Could you check a few things on this model? Use its own coordinates, in mm. A direction names the side the tool comes from. Coordinates: 2 decimals unless noted, no trailing zeros. Order: outer loops, then holes, each group sorted by start corner. A loop starts at its lowest first (then second) coordinate and runs counter-clockwise, first axis right, second up. Notation, with made-up numbers: (9.25, 65.25) - (27.25, 65.25) arc R33 cw to (27.25, 98.25) - close; hole circle Ø7 at (-14.5, 74). An arc over 180 degrees is marked (long way). Answer as a JSON object with one key per item and string values. Group by question number.
(1) Will these pins go through, and if not, where does the flat tip stop? P1, Ø2, axis at x = -14.5, y = 11.5, coming from the +Z side; P2, Ø5, axis at x = 33.5, z = 35.5, coming from the +Y side; P3, Ø7, axis at x = -33.5, z = -33.5, coming from the -Y side.
(2) We'd pull the mould along X, two halves only. Please class faces 4 (the flat face through (-1, 4, 42.5)), 5 (the flat face through (-42.5, 4, 1)), 6 (the flat face through (36.1, 4.166, -34.3)): pulls with the +X half, pulls with the -X half, needs draft (parallel to the pull), parting line crosses it, or undercut.
(3) Imagine slicing it at B-B, the plane x = -33.5. Write out the boundary of the cut face in (y, z), and give its area (3 significant figures).
(4) Please list where these lines run through material, in increasing order: probe 1 along Z at (x, y) = (33.5, 7); probe 2 along Z at (x, y) = (33.5, 8.25).
(5) Imagine slicing it at A-A, the plane z = 33.5. Write out the boundary of the cut face in (x, y), and give its area (3 significant figures).
(6) Which directions (+Z, -Z, +X, -X, +Y, -Y) give clear straight access to the entire face, cutting with the end or side of a thin tool? Please do faces 1 (the flat face through (-14.5, 4, -40)), 2 (the flat face through (-32.7, 4.166, 30.9)), 3 (the flat face through (0, 10, -15)).
from build123d import *

# Parameters (mm, degrees)
SKETCH1_W           = 85
SKETCH1_H           = 85
SKETCH1_R           = 2.4575
BOSS_EXTRUDE1_DEPTH = 8
SKETCH2_R           = 3.969
CUT_EXTRUDE1_DEPTH  = 4.166
SKETCH3_R           = 5
SKETCH3_R_2         = 2.4575
BOSS_EXTRUDE2_DEPTH = 3.5
BOSS_EXTRUDE3_DEPTH = 5
SKETCH5_W           = 29
SKETCH5_H           = 8
CUT_EXTRUDE2_DEPTH  = 10
FILLET1_R           = 2.5
CUT_EXTRUDE3_REACH  = 59.5


with BuildPart() as part:
    # Sketch1 → Boss-Extrude1 (new body)
    with BuildSketch(Plane(origin=(0, 0, 0), x_dir=(1, 0, 0), z_dir=(0, 1, 0))):
        Rectangle(SKETCH1_W, SKETCH1_H)
        with Locations((-33.5, 33.5)):
            Circle(SKETCH1_R, mode=Mode.SUBTRACT)
        with Locations((-33.5, -33.5)):
            Circle(SKETCH1_R, mode=Mode.SUBTRACT)
        with Locations((33.5, -33.5)):
            Circle(SKETCH1_R, mode=Mode.SUBTRACT)
        with Locations((33.5, 33.5)):
            Circle(SKETCH1_R, mode=Mode.SUBTRACT)
    extrude(amount=BOSS_EXTRUDE1_DEPTH)

    # Sketch2 → Cut-Extrude1 (cut)
    with BuildSketch(Plane.XZ):
        with Locations((-33.5, 33.5)):
            Circle(SKETCH2_R)
        with Locations((33.5, 33.5)):
            Circle(SKETCH2_R)
        with Locations((33.5, -33.5)):
            Circle(SKETCH2_R)
        with Locations((-33.5, -33.5)):
            Circle(SKETCH2_R)
    extrude(amount=-CUT_EXTRUDE1_DEPTH, mode=Mode.SUBTRACT)

    # Sketch3 → Boss-Extrude2 (add)
    with BuildSketch(Plane(origin=(0, 8, 0), x_dir=(1, 0, 0), z_dir=(0, 1, 0))):
        with Locations((33.5, -33.5)):
            Circle(SKETCH3_R)
        with Locations((33.5, -33.5)):
            Circle(SKETCH3_R_2, mode=Mode.SUBTRACT)
        with Locations((-33.5, -33.5)):
            Circle(SKETCH3_R)
        with Locations((-33.5, -33.5)):
            Circle(SKETCH3_R_2, mode=Mode.SUBTRACT)
        with Locations((-33.5, 33.5)):
            Circle(SKETCH3_R)
        with Locations((-33.5, 33.5)):
            Circle(SKETCH3_R_2, mode=Mode.SUBTRACT)
        with Locations((33.5, 33.5)):
            Circle(SKETCH3_R)
        with Locations((33.5, 33.5)):
            Circle(SKETCH3_R_2, mode=Mode.SUBTRACT)
    extrude(amount=BOSS_EXTRUDE2_DEPTH)

    # Sketch4 → Boss-Extrude3 (add)
    with BuildSketch(Plane(origin=(0, 8, 0), x_dir=(1, 0, 0), z_dir=(0, 1, 0))):
        with BuildLine():
            Line((2.2929, -14.5), (2.2929, -13.7071))
            ThreePointArc((2.2929, -13.7071), (2.000006781, -12.999993219), (1.2929, -12.7071))
            Line((1.2929, -12.7071), (-1.2929, -12.7071))
            ThreePointArc((-1.2929, -12.7071), (-2.000006781, -12.999993219), (-2.2929, -13.7071))
            Line((-2.2929, -13.7071), (-2.2929, -14.5))
            ThreePointArc((-2.2929, -14.5), (-2.439346609, -14.853553391), (-2.7929, -15))
            Line((-2.7929, -15), (-14.5, -15))
            ThreePointArc((-14.5, -15), (-14.853553391, -14.853553391), (-15, -14.5))
            Line((-15, -14.5), (-15, 14.5))
            ThreePointArc((-15, 14.5), (-14.853553391, 14.853553391), (-14.5, 15))
            Line((-14.5, 15), (14.5, 15))
            ThreePointArc((14.5, 15), (14.853553391, 14.853553391), (15, 14.5))
            Line((15, 14.5), (15, -14.5))
            ThreePointArc((15, -14.5), (14.853553391, -14.853553391), (14.5, -15))
            Line((14.5, -15), (2.7929, -15))
            ThreePointArc((2.7929, -15), (2.439346609, -14.853553391), (2.2929, -14.5))
        make_face()
    extrude(amount=BOSS_EXTRUDE3_DEPTH)

    # Sketch5 → Cut-Extrude2 (cut)
    with BuildSketch(Plane(origin=(0, 8, 0), x_dir=(1, 0, 0), z_dir=(0, 1, 0))):
        with Locations((0, 38.5)):
            Rectangle(SKETCH5_W, SKETCH5_H)
    extrude(amount=-CUT_EXTRUDE2_DEPTH, mode=Mode.SUBTRACT)

    # Fillet1
    fillet1_edges = [part.edges().sort_by_distance(p)[0] for p in [
        (14.5, 4, -34.5),
        (-14.5, 4, -34.5),
    ]]
    fillet(fillet1_edges, radius=FILLET1_R)

    # Sketch7 → Cut-Extrude3 (cut, up to next)
    with BuildSketch(Plane(origin=(0, 0, -15), x_dir=(-1, 0, 0), z_dir=(0, 0, -1)), mode=Mode.PRIVATE) as cut_extrude3_sk1:
        Polygon((-14.5, 13), (-14.125, 12.38), (-13.75, 13), align=None)
    cut_extrude3_tool1 = extrude(cut_extrude3_sk1.sketch, amount=-CUT_EXTRUDE3_REACH, mode=Mode.PRIVATE) & part.part
    add(cut_extrude3_tool1.solids().sort_by_distance((14.125, 12.793333, -15))[0], mode=Mode.SUBTRACT)
    # Sketch7 → Cut-Extrude3 (cut, up to next)
    with BuildSketch(Plane(origin=(0, 0, -15), x_dir=(-1, 0, 0), z_dir=(0, 0, -1)), mode=Mode.PRIVATE) as cut_extrude3_sk2:
        Polygon((-12.5, 13), (-12.125, 12.38), (-11.75, 13), align=None)
    cut_extrude3_tool2 = extrude(cut_extrude3_sk2.sketch, amount=-CUT_EXTRUDE3_REACH, mode=Mode.PRIVATE) & part.part
    add(cut_extrude3_tool2.solids().sort_by_distance((12.125, 12.793333, -15))[0], mode=Mode.SUBTRACT)
    # Sketch7 → Cut-Extrude3 (cut, up to next)
    with BuildSketch(Plane(origin=(0, 0, -15), x_dir=(-1, 0, 0), z_dir=(0, 0, -1)), mode=Mode.PRIVATE) as cut_extrude3_sk3:
        Polygon((-10.5, 13), (-10.125, 12.38), (-9.75, 13), align=None)
    cut_extrude3_tool3 = extrude(cut_extrude3_sk3.sketch, amount=-CUT_EXTRUDE3_REACH, mode=Mode.PRIVATE) & part.part
    add(cut_extrude3_tool3.solids().sort_by_distance((10.125, 12.793333, -15))[0], mode=Mode.SUBTRACT)
    # Sketch7 → Cut-Extrude3 (cut, up to next)
    with BuildSketch(Plane(origin=(0, 0, -15), x_dir=(-1, 0, 0), z_dir=(0, 0, -1)), mode=Mode.PRIVATE) as cut_extrude3_sk4:
        Polygon((-8.5, 13), (-8.125, 12.38), (-7.75, 13), align=None)
    cut_extrude3_tool4 = extrude(cut_extrude3_sk4.sketch, amount=-CUT_EXTRUDE3_REACH, mode=Mode.PRIVATE) & part.part
    add(cut_extrude3_tool4.solids().sort_by_distance((8.125, 12.793333, -15))[0], mode=Mode.SUBTRACT)
    # Sketch7 → Cut-Extrude3 (cut, up to next)
    with BuildSketch(Plane(origin=(0, 0, -15), x_dir=(-1, 0, 0), z_dir=(0, 0, -1)), mode=Mode.PRIVATE) as cut_extrude3_sk5:
        Polygon((-6.5, 13), (-6.125, 12.38), (-5.75, 13), align=None)
    cut_extrude3_tool5 = extrude(cut_extrude3_sk5.sketch, amount=-CUT_EXTRUDE3_REACH, mode=Mode.PRIVATE) & part.part
    add(cut_extrude3_tool5.solids().sort_by_distance((6.125, 12.793333, -15))[0], mode=Mode.SUBTRACT)
    # Sketch7 → Cut-Extrude3 (cut, up to next)
    with BuildSketch(Plane(origin=(0, 0, -15), x_dir=(-1, 0, 0), z_dir=(0, 0, -1)), mode=Mode.PRIVATE) as cut_extrude3_sk6:
        Polygon((-4.5, 13), (-4.125, 12.38), (-3.75, 13), align=None)
    cut_extrude3_tool6 = extrude(cut_extrude3_sk6.sketch, amount=-CUT_EXTRUDE3_REACH, mode=Mode.PRIVATE) & part.part
    add(cut_extrude3_tool6.solids().sort_by_distance((4.125, 12.793333, -15))[0], mode=Mode.SUBTRACT)
    # Sketch7 → Cut-Extrude3 (cut, up to next)
    with BuildSketch(Plane(origin=(0, 0, -15), x_dir=(-1, 0, 0), z_dir=(0, 0, -1)), mode=Mode.PRIVATE) as cut_extrude3_sk7:
        Polygon((-2.5, 13), (-2.125, 12.38), (-1.75, 13), align=None)
    cut_extrude3_tool7 = extrude(cut_extrude3_sk7.sketch, amount=-CUT_EXTRUDE3_REACH, mode=Mode.PRIVATE) & part.part
    add(cut_extrude3_tool7.solids().sort_by_distance((2.125, 12.793333, -15))[0], mode=Mode.SUBTRACT)
    # Sketch7 → Cut-Extrude3 (cut, up to next)
    with BuildSketch(Plane(origin=(0, 0, -15), x_dir=(-1, 0, 0), z_dir=(0, 0, -1)), mode=Mode.PRIVATE) as cut_extrude3_sk8:
        Polygon((-0.5, 13), (-0.125, 12.38), (0.25, 13), align=None)
    cut_extrude3_tool8 = extrude(cut_extrude3_sk8.sketch, amount=-CUT_EXTRUDE3_REACH, mode=Mode.PRIVATE) & part.part
    add(cut_extrude3_tool8.solids().sort_by_distance((0.125, 12.793333, -15))[0], mode=Mode.SUBTRACT)
    # Sketch7 → Cut-Extrude3 (cut, up to next)
    with BuildSketch(Plane(origin=(0, 0, -15), x_dir=(-1, 0, 0), z_dir=(0, 0, -1)), mode=Mode.PRIVATE) as cut_extrude3_sk9:
        Polygon((1.5, 13), (1.875, 12.38), (2.25, 13), align=None)
    cut_extrude3_tool9 = extrude(cut_extrude3_sk9.sketch, amount=-CUT_EXTRUDE3_REACH, mode=Mode.PRIVATE) & part.part
    add(cut_extrude3_tool9.solids().sort_by_distance((-1.875, 12.793333, -15))[0], mode=Mode.SUBTRACT)
    # Sketch7 → Cut-Extrude3 (cut, up to next)
    with BuildSketch(Plane(origin=(0, 0, -15), x_dir=(-1, 0, 0), z_dir=(0, 0, -1)), mode=Mode.PRIVATE) as cut_extrude3_sk10:
        Polygon((3.5, 13), (3.875, 12.38), (4.25, 13), align=None)
    cut_extrude3_tool10 = extrude(cut_extrude3_sk10.sketch, amount=-CUT_EXTRUDE3_REACH, mode=Mode.PRIVATE) & part.part
    add(cut_extrude3_tool10.solids().sort_by_distance((-3.875, 12.793333, -15))[0], mode=Mode.SUBTRACT)
    # Sketch7 → Cut-Extrude3 (cut, up to next)
    with BuildSketch(Plane(origin=(0, 0, -15), x_dir=(-1, 0, 0), z_dir=(0, 0, -1)), mode=Mode.PRIVATE) as cut_extrude3_sk11:
        Polygon((5.5, 13), (5.875, 12.38), (6.25, 13), align=None)
    cut_extrude3_tool11 = extrude(cut_extrude3_sk11.sketch, amount=-CUT_EXTRUDE3_REACH, mode=Mode.PRIVATE) & part.part
    add(cut_extrude3_tool11.solids().sort_by_distance((-5.875, 12.793333, -15))[0], mode=Mode.SUBTRACT)
    # Sketch7 → Cut-Extrude3 (cut, up to next)
    with BuildSketch(Plane(origin=(0, 0, -15), x_dir=(-1, 0, 0), z_dir=(0, 0, -1)), mode=Mode.PRIVATE) as cut_extrude3_sk12:
        Polygon((7.5, 13), (7.875, 12.38), (8.25, 13), align=None)
    cut_extrude3_tool12 = extrude(cut_extrude3_sk12.sketch, amount=-CUT_EXTRUDE3_REACH, mode=Mode.PRIVATE) & part.part
    add(cut_extrude3_tool12.solids().sort_by_distance((-7.875, 12.793333, -15))[0], mode=Mode.SUBTRACT)
    # Sketch7 → Cut-Extrude3 (cut, up to next)
    with BuildSketch(Plane(origin=(0, 0, -15), x_dir=(-1, 0, 0), z_dir=(0, 0, -1)), mode=Mode.PRIVATE) as cut_extrude3_sk13:
        Polygon((9.5, 13), (9.875, 12.38), (10.25, 13), align=None)
    cut_extrude3_tool13 = extrude(cut_extrude3_sk13.sketch, amount=-CUT_EXTRUDE3_REACH, mode=Mode.PRIVATE) & part.part
    add(cut_extrude3_tool13.solids().sort_by_distance((-9.875, 12.793333, -15))[0], mode=Mode.SUBTRACT)
    # Sketch7 → Cut-Extrude3 (cut, up to next)
    with BuildSketch(Plane(origin=(0, 0, -15), x_dir=(-1, 0, 0), z_dir=(0, 0, -1)), mode=Mode.PRIVATE) as cut_extrude3_sk14:
        Polygon((11.5, 13), (11.875, 12.38), (12.25, 13), align=None)
    cut_extrude3_tool14 = extrude(cut_extrude3_sk14.sketch, amount=-CUT_EXTRUDE3_REACH, mode=Mode.PRIVATE) & part.part
    add(cut_extrude3_tool14.solids().sort_by_distance((-11.875, 12.793333, -15))[0], mode=Mode.SUBTRACT)
    # Sketch7 → Cut-Extrude3 (cut, up to next)
    with BuildSketch(Plane(origin=(0, 0, -15), x_dir=(-1, 0, 0), z_dir=(0, 0, -1)), mode=Mode.PRIVATE) as cut_extrude3_sk15:
        Polygon((13.5, 13), (13.875, 12.38), (14.25, 13), align=None)
    cut_extrude3_tool15 = extrude(cut_extrude3_sk15.sketch, amount=-CUT_EXTRUDE3_REACH, mode=Mode.PRIVATE) & part.part
    add(cut_extrude3_tool15.solids().sort_by_distance((-13.875, 12.793333, -15))[0], mode=Mode.SUBTRACT)


solid = part.part
Result set:
{
 "1": {"P1": "stops at z = 15", "P2": "stops at y = 11.5", "P3": "stops at y = 4.17"},
 "2": {"face 4": "needs draft", "face 5": "pulls with the -X half", "face 6": "undercut"},
 "3": {"outline": "(0, -42.5) - (8, -42.5) - (8, -38.5) - (11.5, -38.5) - (11.5, -35.96) - (4.17, -35.96) - (4.17, -37.47) - (0, -37.47) - close; (0, -29.53) - (4.17, -29.53) - (4.17, -31.04) - (11.5, -31.04) - (11.5, -28.5) - (8, -28.5) - (8, 28.5) - (11.5, 28.5) - (11.5, 31.04) - (4.17, 31.04) - (4.17, 29.53) - (0, 29.53) - close; (0, 37.47) - (4.17, 37.47) - (4.17, 35.96) - (11.5, 35.96) - (11.5, 38.5) - (8, 38.5) - (8, 42.5) - (0, 42.5) - close", "area": "612 mm^2"},
 "4": {"probe 1": "z = -42.5 to -35.96, -31.04 to 31.04, 35.96 to 42.5", "probe 2": "z = -38.5 to -35.96, -31.04 to -28.5, 28.5 to 31.04, 35.96 to 38.5"},
 "5": {"outline": "(-42.5, 0) - (-37.47, 0) - (-37.47, 4.17) - (-35.96, 4.17) - (-35.96, 11.5) - (-38.5, 11.5) - (-38.5, 8) - (-42.5, 8) - close; (-31.04, 4.17) - (-29.53, 4.17) - (-29.53, 0) - (29.53, 0) - (29.53, 4.17) - (31.04, 4.17) - (31.04, 11.5) - (28.5, 11.5) - (28.5, 8) - (-28.5, 8) - (-28.5, 11.5) - (-31.04, 11.5) - close; (35.96, 4.17) - (37.47, 4.17) - (37.47, 0) - (42.5, 0) - (42.5, 8) - (38.5, 8) - (38.5, 11.5) - (35.96, 11.5) - close", "area": "612 mm^2"},
 "6": {"face 1": "-Z, +Y, -Y", "face 2": "-Y", "face 3": "-Z, +X, -X, +Y"}
}
